```python
from build123d import *

# Parameters (mm, degrees)
F0_W    = 1.85
F0_H    = 5
F3_SIZE = 1


# Not quite as in the source:
# - a fillet or chamfer that OpenCascade refuses, or shapes differently, is made with other operations: its cross-section is extruded or revolved along the edge and cut away or added


with BuildPart() as f1:
    # F0 (on Right) → F1 (revolve)
    with BuildSketch(Plane.YZ):
        with Locations((1.6295755848, 1.9221331838)):
            Rectangle(F0_W, F0_H)
        Polygon((2.5545755848, 7.4221331838), (2.5545755848, 4.4221331838), (2.5545755848, -0.5778668162), (2.5545755848, -3.5778668162), (4.5545755848, -3.5778668162), (4.5545755848, -0.5778668162), (8.5545755848, -0.5778668162), (8.5545755848, 4.4221331838), (4.5545755848, 4.4221331838), (4.5545755848, 7.4221331838), align=None)
    revolve(axis=Axis((0, -7.4454244152, 1.9221331838), (0, 0, -1)))

    # F2: fillet of radius 3 on 2 edges, made by hand

    # F2_s1 → F2_t2 (revolve)
    with BuildSketch(Plane.YZ):
        with BuildLine():
            ThreePointArc((0.7045755848, 4.4221331838), (2.0495705748, 5.5271302594), (2.5545755848, 7.1929633843))
            Line((2.5545755848, 7.1929633843), (2.5545755848, 4.4221331838))
            Line((2.5545755848, 4.4221331838), (0.7045755848, 4.4221331838))
        make_face()
    revolve(axis=Axis((0, -7.4454244152, 4.4221331838), (0, 0, -1)))

    # F2_s3 → F2_t4 (revolve)
    with BuildSketch(Plane.YZ):
        with BuildLine():
            ThreePointArc((0.7045755848, -0.5778668162), (2.0495705748, -1.6828638918), (2.5545755848, -3.3486970167))
            Line((2.5545755848, -3.3486970167), (2.5545755848, -0.5778668162))
            Line((2.5545755848, -0.5778668162), (0.7045755848, -0.5778668162))
        make_face()
    revolve(axis=Axis((0, -7.4454244152, -0.5778668162), (0, 0, -1)))

    # F3
    f3_edges = [f1.edges().sort_by_distance(p)[0] for p in [
        (0, -23.445424, -0.577867),
        (0, -23.445424, 4.422133),
    ]]
    chamfer(f3_edges, length=F3_SIZE)


solid = f1.part
```
The model under review builds one solid part; all positions refer to its coordinate system, in mm. A direction names the side the tool comes from. Coordinates: 2 decimals unless noted, no trailing zeros. Loops run counter-clockwise (first coordinate to the right, second up) from the corner with the lowest first, then second, coordinate; pieces in that order, holes last. Notation, with made-up numbers: (6.25, 79.5) -> (56.25, 79.5) arc R30 cw to (56.25, 112.5) -> close; hole circle Ø7 at (7.5, -21). An arc over 180 degrees is marked (long way). Answer as CSV lines item,"result".
Item 1: Draft analysis for pull direction Y (two halves, no side actions). For faces 1 (the cylindrical face through (-4.96, -13.91, 1.96)), 2 (the flat face through (12.3, -7.4, -0.578)), 3 (the cylindrical face through (3.6, 4, 5.9)), state which applies: +Y half, -Y half, draft (parallel to the pull), parting line (faces both ways), or undercut.
Results below:
face 1,"undercut"
face 2,"draft"
face 3,"parting line"
Item 2: Machinability: for faces 4 (the flat face through (10.1, -14.2, 4.422)), 5 (the cylindrical face through (3.6, 4, -2.1)), 6 (the flat face through (10, -10, 7.422)), which of the approach directions +Z, -Z, +X, -X, +Y, -Y give a long, thin tool a straight path to every point of the face, cutting with its end or side? Answer none if there is none.
Results below:
face 4,"+Z"
face 5,"-Z"
face 6,"+Z, +X, -X, +Y, -Y"
Item 3: Take a section at C-C, the plane z = 6.75. State the section outline as (x, y) points.
Results below:
outline,"circle Ø24 at (0, -7.45); hole circle Ø19.93 at (0, -7.45)"
Item 4: Insertion check: pin 1 (3 mm diameter, centred on x = 10, z = 0.5, fed in from +Y); pin 2 (5 mm diameter, centred on y = -3, z = -1.5, fed in from +X); pin 3 (8 mm diameter, centred on x = 3.5, y = -12, fed in from +Z). Each pin has a flat end and moves straight along its axis. Give the tip position at first contact, or say it passes through.
Results below:
pin 1,"stops at y = 6.11"
pin 2,"stops at x = 15.74"
pin 3,"stops at z = 5.98"
Item 5: For L1, parallel to Z at x = -7, y = 4; L2, parallel to X at y = -7, z = 1.25; L3, parallel to Y at x = -5.5, z = 6, list the stretches that pass through material, from the lowest coordinate up.
Results below:
L1,"z = -0.58 to 4.42"
L2,"x = -15.99 to -8.14, 8.14 to 15.99"
L3,"y = -18.11 to -15.5, 0.61 to 3.22"
Item 6: Take a section at A-A, the plane x = 0. State the section outline as (y, z) points.
Results below:
outline,"(-23.45, 0.42) -> (-22.45, -0.58) -> (-19.45, -0.58) -> (-19.45, -3.58) -> (-17.45, -3.58) -> (-17.45, -3.35) arc R3 cw to (-15.6, -0.58) -> (-15.6, 4.42) arc R3 cw to (-17.45, 7.19) -> (-17.45, 7.42) -> (-19.45, 7.42) -> (-19.45, 4.42) -> (-22.45, 4.42) -> (-23.45, 3.42) -> close; (0.7, -0.58) arc R3 cw to (2.55, -3.35) -> (2.55, -3.58) -> (4.55, -3.58) -> (4.55, -0.58) -> (7.55, -0.58) -> (8.55, 0.42) -> (8.55, 3.42) -> (7.55, 4.42) -> (4.55, 4.42) -> (4.55, 7.42) -> (2.55, 7.42) -> (2.55, 7.19) arc R3 cw to (0.7, 4.42) -> close"
Item 7: Take a section at B-B, the plane z = 1. State the section outline as (x, y) points, and give its area (3 significant figures).
Results below:
outline,"circle Ø32 at (0, -7.45); hole circle Ø16.3 at (0, -7.45)"
area,"596 mm2"
